The model under review builds one solid part; all positions refer to its coordinate system, in mm. A direction names the side the tool comes from. Coordinates: 2 decimals unless noted, no trailing zeros. Write each loop counter-clockwise with the first axis right and the second up, starting at its lowest first coordinate (ties: lowest second). Pieces come first, ordered by that corner, then holes.
```python
from build123d import *

# Parameters (mm, degrees)
SKETCH_2_R      = 1.65
EXTRUDE_1_DEPTH = 3
FILLET_3_R      = 2.5
FILLET_3_2_R    = 5


with BuildPart() as part:
    # Sketch 2 → Extrude 1 (new body)
    with BuildSketch(Plane.XY):
        with BuildLine():
            Line((-8.45, -27.5), (8.45, -27.5))
            Line((8.45, -27.5), (8.45, -14.7))
            ThreePointArc((8.45, -14.7), (7.35, -13.6), (8.45, -12.5))
            Line((8.45, -12.5), (10, -12.5))
            Line((10, -12.5), (10, 10))
            Line((10, 10), (-10, 10))
            Line((-10, 10), (-10, -12.5))
            Line((-10, -12.5), (-8.45, -12.5))
            ThreePointArc((-8.45, -12.5), (-7.35, -13.6), (-8.45, -14.7))
            Line((-8.45, -14.7), (-8.45, -27.5))
        make_face()
        with Locations((-4.9, 5)):
            Circle(SKETCH_2_R, mode=Mode.SUBTRACT)
        with Locations((-4.9, -5)):
            Circle(SKETCH_2_R, mode=Mode.SUBTRACT)
        with Locations((4.9, -5)):
            Circle(SKETCH_2_R, mode=Mode.SUBTRACT)
        with Locations((4.9, 5)):
            Circle(SKETCH_2_R, mode=Mode.SUBTRACT)
        with Locations((0, -20)):
            Circle(SKETCH_2_R, mode=Mode.SUBTRACT)
    extrude(amount=EXTRUDE_1_DEPTH)

    # Fillet 3
    fillet_3_edges = [part.edges().sort_by_distance(p)[0] for p in [
        (-8.45, -27.5, 1.5),
        (8.45, -27.5, 1.5),
    ]]
    fillet(fillet_3_edges, radius=FILLET_3_R)

    # Fillet 3 2
    fillet_3_2_edges = [part.edges().sort_by_distance(p)[0] for p in [
        (10, 10, 1.5),
        (-10, 10, 1.5),
    ]]
    fillet(fillet_3_2_edges, radius=FILLET_3_2_R)


solid = part.part
```
Item 1: Take a section at A-A, the plane y = -20. Write out the cut boundary in (x, z), plus the area to 3 significant figures.
Solved:
outline: (-8.45, 0) - (-1.65, 0) - (-1.65, 3) - (-8.45, 3) - close; (1.65, 0) - (8.45, 0) - (8.45, 3) - (1.65, 3) - close
area: 40.8 mm2
Item 2: Take a section at C-C, the plane y = -5. Write out the cut boundary in (x, z), plus the area to 3 significant figures.
Solved:
outline: (-10, 0) - (-6.55, 0) - (-6.55, 3) - (-10, 3) - close; (-3.25, 0) - (3.25, 0) - (3.25, 3) - (-3.25, 3) - close; (6.55, 0) - (10, 0) - (10, 3) - (6.55, 3) - close
area: 40.2 mm2
Item 3: Take a section at D-D, the plane x = 1. Write out the cut boundary in (y, z).
Solved:
outline: (-27.5, 0) - (-21.31, 0) - (-21.31, 3) - (-27.5, 3) - close; (-18.69, 0) - (10, 0) - (10, 3) - (-18.69, 3) - close
Item 4: Take a section at B-B, the plane z = 2.25. Write out the cut boundary in (x, y), plus the area to 3 significant figures.
Solved:
outline: (-10, -12.5) - (-8.45, -12.5) arc R1.1 cw to (-8.45, -14.7) - (-8.45, -25) arc R2.5 ccw to (-5.95, -27.5) - (5.95, -27.5) arc R2.5 ccw to (8.45, -25) - (8.45, -14.7) arc R1.1 cw to (8.45, -12.5) - (10, -12.5) - (10, 5) arc R5 ccw to (5, 10) - (-5, 10) arc R5 ccw to (-10, 5) - close; hole circle Ø3.3 at (-4.9, -5); hole circle Ø3.3 at (-4.9, 5); hole circle Ø3.3 at (0, -20); hole circle Ø3.3 at (4.9, -5); hole circle Ø3.3 at (4.9, 5)
area: 644 mm2
Item 5: To check wall thickness, follow line 1 along Y through (x, z) = (-4.9, 0.95); line 2 along Y through (x, z) = (4, 0.8); line 3 along X through (y, z) = (4, 1). State the ranges of each line that lie inside material, in increasing order.
Solved:
line 1: y = -27.5 to -6.65, -3.35 to 3.35, 6.65 to 10
line 2: y = -27.5 to -6.38, -3.62 to 3.62, 6.38 to 10
line 3: x = -10 to -6.21, -3.59 to 3.59, 6.21 to 10
Item 6: Machinability: for faces 5 (the face through (-9, -12.5, 1)), 6 (the face through (0, 10, 1)), which of the approach directions +Z, -Z, +X, -X, +Y, -Y give a long, thin tool a straight path to every point of the face, cutting with its end or side? Answer none if there is none.
Solved:
face 5: +Z, -Z, -X, -Y
face 6: +Z, -Z, +X, -X, +Y
Item 7: Mouldability with a two-part tool opening along X and no side actions: class faces 1 (the face through (-7.698, -26.787, 1.521)), 2 (the face through (4.5, 3.4, 1.5)), 3 (the face through (-3.376, -5.632, 1.479)), 4 (the face through (9, -12.5, 1)) as pulls with the +X half, pulls with the -X half, needs draft (parallel to the pull), parting line crosses it, or undercut.
Solved:
face 1: pulls with the -X half
face 2: undercut
face 3: undercut
face 4: needs draft
Item 8: For pin 1 (0.8 mm diameter, centred on x = 9.5, z = 1.5, fed in from -Y); pin 2 (1.5 mm diameter, centred on y = -14, z = 2, fed in from -X); pin 3 (2.5 mm diameter, centred on x = 0, y = -20, fed in from +Z); pin 4 (1.7 mm diameter, centred on x = -9, z = 1, fed in from -Y), all flat-tipped, find the tip position at first contact; note any pin that passes through.
Solved:
pin 1: stops at y = -12.5
pin 2: stops at x = -8.45
pin 3: passes through
pin 4: stops at y = -26.19
